Geometry: final body of the model. Coordinates: model frame, mm. Face numbers are marked on the shaded views. A direction names the side the tool comes from. Round coordinates to 2 decimals unless told otherwise and drop trailing zeros. Loops run counter-clockwise (first coordinate to the right, second up) from the corner with the lowest first, then second, coordinate; pieces in that order, holes last. Notation, with made-up numbers: (76.25, 88) - (127.25, 88) arc R26 ccw to (127.25, 120) - close; hole circle Ø9 at (0.5, 87). An arc over 180 degrees is marked (long way). Answer as a JSON object with one key per item and string values. Group by question number.
Item 1: Reachability of the marked faces 1, 2, 3, 4 and 5 from +Z, -Z, +X, -X, +Y, -Y: full face, straight path, thin tool, end or side. Return the list, or none.
Item 2: Draft query along X for the marked faces 6, 7 and 8. Return one class per face: released by +X, released by -X, zero draft, split by the parting line, or undercut.
Item 3: Section D-D (z = 1). Return the cut outline in (x, y).
Item 4: Section B-B (y = 13). Return the cut outline in (x, z), plus the area to 3 significant figures.
Item 5: Line query: line 1 (Y direction, x = 16, z = 5); line 2 (Y direction, x = 2, z = 3); line 3 (Y direction, x = -2, z = 9.75). Output: solid intervals per line, ascending.
Item 6: First-contact query: pin 1 (3.5 mm diameter, centred on x = -15.88, y = 15.88, fed in from +Z); pin 2 (12 mm diameter, centred on x = -3.5, y = 9, fed in from -Z); pin 3 (4 mm diameter, centred on x = -3, y = -0.5, fed in from -Z). Flat tips, straight axial feed; report the tip coordinate or a pass-through.
Item 7: Section A-A (z = 9). Return the cut outline in (x, y).
Item 8: Section C-C (x = -12.5). Return the cut outline in (y, z), plus the area to 3 significant figures.
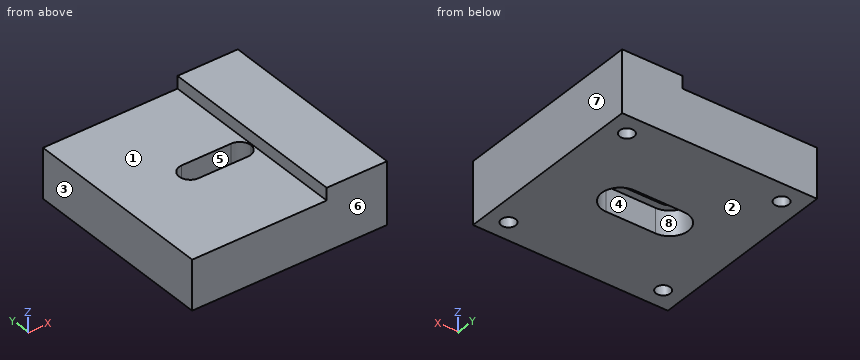
```python
from build123d import *

# Parameters (mm, degrees)
F0_W     = 27.6225
F0_H     = 40.005
F0_R     = 3.302
F0_W_2   = 12.3825
F0_R_2   = 2.159
F1_DEPTH = 10.16
F2_DEPTH = 12.7
F4_DEPTH = 25.4
F5_DEPTH = 5.08
F6_DEPTH = 12.7
F8_D     = 2.9464
F8_DEPTH = 7.62
F8_TIP   = 0.885187864


# Not quite as in the source:
# - a feature names something its author has since deleted; it is built from what else it names


with BuildPart() as f1:
    # F0 (on Top) → F1 (new body)
    with BuildSketch(Plane.XY):
        with Locations((-6.19125, 0)):
            Rectangle(F0_W, F0_H)
        with Locations((-15.875, -15.875)):
            Circle(F0_R, mode=Mode.SUBTRACT)
        with Locations((-15.875, 15.875)):
            Circle(F0_R, mode=Mode.SUBTRACT)
        with Locations((13.81125, 0)):
            Rectangle(F0_W_2, F0_H)
        with Locations((15.875, -15.875)):
            Circle(F0_R, mode=Mode.SUBTRACT)
        with Locations((15.875, 15.875)):
            Circle(F0_R, mode=Mode.SUBTRACT)
        with Locations((-15.875, 15.875)):
            Circle(F0_R)
        with Locations((-15.875, 15.875)):
            Circle(F0_R_2, mode=Mode.SUBTRACT)
        with Locations((15.875, 15.875)):
            Circle(F0_R)
        with Locations((15.875, 15.875)):
            Circle(F0_R_2, mode=Mode.SUBTRACT)
        with Locations((15.875, -15.875)):
            Circle(F0_R)
        with Locations((15.875, -15.875)):
            Circle(F0_R_2, mode=Mode.SUBTRACT)
        with Locations((-15.875, -15.875)):
            Circle(F0_R)
        with Locations((-15.875, -15.875)):
            Circle(F0_R_2, mode=Mode.SUBTRACT)
        with Locations((-15.875, 15.875)):
            Circle(F0_R_2)
        with Locations((15.875, 15.875)):
            Circle(F0_R_2)
        with Locations((15.875, -15.875)):
            Circle(F0_R_2)
        with Locations((-15.875, -15.875)):
            Circle(F0_R_2)
    extrude(amount=F1_DEPTH)

    # F0 (on Top) → F2 (join)
    with BuildSketch(Plane.XY):
        with Locations((13.81125, 0)):
            Rectangle(F0_W_2, F0_H)
        with Locations((15.875, -15.875)):
            Circle(F0_R, mode=Mode.SUBTRACT)
        with Locations((15.875, 15.875)):
            Circle(F0_R, mode=Mode.SUBTRACT)
    extrude(amount=F2_DEPTH)

    # F3 (on face) → F4 (cut)
    with BuildSketch(Plane(origin=(0, 0, 0), x_dir=(1, 0, 0), z_dir=(0, 0, -1))):
        with BuildLine():
            ThreePointArc((-2.794, 0), (-3.4635538982, 1.6164461018), (-5.08, 2.286))
            ThreePointArc((-5.08, 2.286), (-7.366, 0), (-5.08, -2.286))
            ThreePointArc((-5.08, -2.286), (-3.4635538982, -1.6164461018), (-2.794, 0))
        make_face()
        with BuildLine():
            ThreePointArc((7.366, 0), (6.6964461018, 1.6164461018), (5.08, 2.286))
            ThreePointArc((5.08, 2.286), (2.794, 0), (5.08, -2.286))
            ThreePointArc((5.08, -2.286), (6.6964461018, -1.6164461018), (7.366, 0))
        make_face()
        with BuildLine():
            ThreePointArc((-1.27, 0), (-1.4655166344, 1.2048277885), (-2.032, 2.286))
            Line((-2.032, 2.286), (-5.08, 2.286))
            ThreePointArc((-5.08, 2.286), (-3.4635538982, 1.6164461018), (-2.794, 0))
            ThreePointArc((-2.794, 0), (-3.4635538982, -1.6164461018), (-5.08, -2.286))
            Line((-5.08, -2.286), (-2.032, -2.286))
            ThreePointArc((-2.032, -2.286), (-1.4655166344, -1.2048277885), (-1.27, 0))
        make_face()
        with BuildLine():
            ThreePointArc((2.032, -2.286), (1.27, 0), (2.032, 2.286))
            Line((2.032, 2.286), (-2.032, 2.286))
            ThreePointArc((-2.032, 2.286), (-1.4655166344, 1.2048277885), (-1.27, 0))
            ThreePointArc((-1.27, 0), (-1.4655166344, -1.2048277885), (-2.032, -2.286))
            Line((-2.032, -2.286), (2.032, -2.286))
        make_face()
        with BuildLine():
            Line((5.08, 2.286), (2.032, 2.286))
            ThreePointArc((2.032, 2.286), (1.27, 0), (2.032, -2.286))
            Line((2.032, -2.286), (5.08, -2.286))
            ThreePointArc((5.08, -2.286), (2.794, 0), (5.08, 2.286))
        make_face()
    extrude(amount=-F4_DEPTH, mode=Mode.SUBTRACT)

    # F3 (on face) → F5 (cut)
    with BuildSketch(Plane(origin=(0, 0, 0), x_dir=(1, 0, 0), z_dir=(0, 0, -1))):
        with BuildLine():
            ThreePointArc((-1.27, 0), (-1.4655166344, 1.2048277885), (-2.032, 2.286))
            Line((-2.032, 2.286), (-5.08, 2.286))
            ThreePointArc((-5.08, 2.286), (-3.4635538982, 1.6164461018), (-2.794, 0))
            ThreePointArc((-2.794, 0), (-3.4635538982, -1.6164461018), (-5.08, -2.286))
            Line((-5.08, -2.286), (-2.032, -2.286))
            ThreePointArc((-2.032, -2.286), (-1.4655166344, -1.2048277885), (-1.27, 0))
        make_face()
        with BuildLine():
            ThreePointArc((-2.032, 2.286), (-3.3761162011, 3.4077675977), (-5.08, 3.81))
            ThreePointArc((-5.08, 3.81), (-8.89, 0), (-5.08, -3.81))
            ThreePointArc((-5.08, -3.81), (-3.3761162011, -3.4077675977), (-2.032, -2.286))
            Line((-2.032, -2.286), (-5.08, -2.286))
            ThreePointArc((-5.08, -2.286), (-7.366, 0), (-5.08, 2.286))
            Line((-5.08, 2.286), (-2.032, 2.286))
        make_face()
        with BuildLine():
            ThreePointArc((2.032, 2.286), (3.3761162011, 3.4077675977), (5.08, 3.81))
            Line((5.08, 3.81), (-5.08, 3.81))
            ThreePointArc((-5.08, 3.81), (-3.3761162011, 3.4077675977), (-2.032, 2.286))
            Line((-2.032, 2.286), (2.032, 2.286))
        make_face()
        with BuildLine():
            ThreePointArc((2.032, -2.286), (1.27, 0), (2.032, 2.286))
            Line((2.032, 2.286), (-2.032, 2.286))
            ThreePointArc((-2.032, 2.286), (-1.4655166344, 1.2048277885), (-1.27, 0))
            ThreePointArc((-1.27, 0), (-1.4655166344, -1.2048277885), (-2.032, -2.286))
            Line((-2.032, -2.286), (2.032, -2.286))
        make_face()
        with BuildLine():
            Line((5.08, 2.286), (2.032, 2.286))
            ThreePointArc((2.032, 2.286), (1.27, 0), (2.032, -2.286))
            Line((2.032, -2.286), (5.08, -2.286))
            ThreePointArc((5.08, -2.286), (2.794, 0), (5.08, 2.286))
        make_face()
        with BuildLine():
            ThreePointArc((5.08, -3.81), (7.7740768363, -2.6940768363), (8.89, 0))
            ThreePointArc((8.89, 0), (7.7740768363, 2.6940768363), (5.08, 3.81))
            ThreePointArc((5.08, 3.81), (3.3761162011, 3.4077675977), (2.032, 2.286))
            Line((2.032, 2.286), (5.08, 2.286))
            ThreePointArc((5.08, 2.286), (6.6964461018, 1.6164461018), (7.366, 0))
            ThreePointArc((7.366, 0), (6.6964461018, -1.6164461018), (5.08, -2.286))
            Line((5.08, -2.286), (2.032, -2.286))
            ThreePointArc((2.032, -2.286), (3.3761162011, -3.4077675977), (5.08, -3.81))
        make_face()
        with BuildLine():
            Line((-5.08, -3.81), (5.08, -3.81))
            ThreePointArc((5.08, -3.81), (3.3761162011, -3.4077675977), (2.032, -2.286))
            Line((2.032, -2.286), (-2.032, -2.286))
            ThreePointArc((-2.032, -2.286), (-3.3761162011, -3.4077675977), (-5.08, -3.81))
        make_face()
    extrude(amount=-F5_DEPTH, mode=Mode.SUBTRACT)

    # F0 (on Top) → F6 (join)
    with BuildSketch(Plane.XY):
        with Locations((15.875, 15.875)):
            Circle(F0_R)
        with Locations((15.875, 15.875)):
            Circle(F0_R_2, mode=Mode.SUBTRACT)
        with Locations((15.875, 15.875)):
            Circle(F0_R_2)
        with Locations((15.875, -15.875)):
            Circle(F0_R)
        with Locations((15.875, -15.875)):
            Circle(F0_R_2, mode=Mode.SUBTRACT)
        with Locations((15.875, -15.875)):
            Circle(F0_R_2)
    extrude(amount=F6_DEPTH)

    # F8
    with Locations(Plane(origin=(0, 0, 0), x_dir=(1, 0, 0), z_dir=(0, 0, -1))):
        with Locations((-15.87754, 15.87754), (15.87754, 15.87754), (15.87754, -15.87754), (-15.87754, -15.87754)):
            Hole(F8_D / 2, depth=F8_DEPTH)
            with Locations((0, 0, -(F8_DEPTH + F8_TIP / 2))):  # 118° drill point
                Cone(0, F8_D / 2, F8_TIP, mode=Mode.SUBTRACT)


solid = f1.part
```
Values:
{
 "1": {"face 1": "+Z, -X, +Y, -Y", "face 2": "-Z, +X, -X, +Y, -Y", "face 3": "+Z, -Z, -X, +Y, -Y", "face 4": "-Z", "face 5": "+Z, -Z"},
 "2": {"face 6": "zero draft", "face 7": "released by +X", "face 8": "undercut"},
 "3": {"outline": "(-20, -20) - (20, -20) - (20, 20) - (-20, 20) - close; hole circle Ø2.95 at (-15.88, -15.88); hole circle Ø2.95 at (-15.88, 15.88); hole (-5.08, -3.81) - (5.08, -3.81) arc R3.81 ccw to (5.08, 3.81) - (-5.08, 3.81) arc R3.81 ccw to start; hole circle Ø2.95 at (15.88, -15.88); hole circle Ø2.95 at (15.88, 15.88)"},
 "4": {"outline": "(-20, 0) - (20, 0) - (20, 12.7) - (7.62, 12.7) - (7.62, 10.16) - (-20, 10.16) - close", "area": "438 mm^2"},
 "5": {"line 1": "y = -20 to -17.35, -14.41 to 14.41, 17.35 to 20", "line 2": "y = -20 to -3.81, 3.81 to 20", "line 3": "y = -20 to -2.29, 2.29 to 20"},
 "6": {"pin 1": "stops at z = 10.16", "pin 2": "stops at z = 0", "pin 3": "stops at z = 5.08"},
 "7": {"outline": "(-20, -20) - (20, -20) - (20, 20) - (-20, 20) - close; hole (-5.08, -2.29) - (5.08, -2.29) arc R2.29 ccw to (5.08, 2.29) - (-5.08, 2.29) arc R2.29 ccw to start"},
 "8": {"outline": "(-20, 0) - (20, 0) - (20, 10.16) - (-20, 10.16) - close", "area": "406 mm^2"}
}
